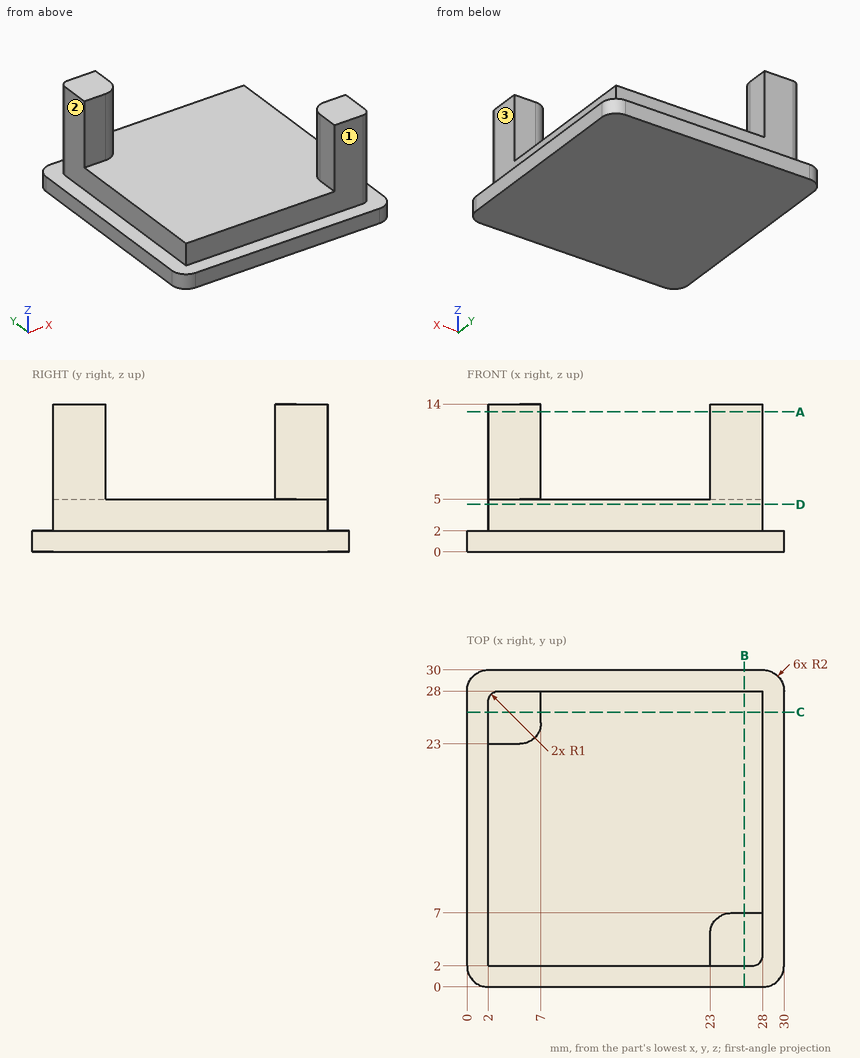
Answer from the drawing. Dimensions are ordinates in mm from the lowest x, y and z of the part. A direction names the side the tool comes from. Round coordinates to 2 decimals unless told otherwise and drop trailing zeros. Loops run counter-clockwise (first coordinate to the right, second up) from the corner with the lowest first, then second, coordinate; pieces in that order, holes last.
(1) For the marked faces 1, 2 and 3, determine the directions among +Z, -Z, +X, -X, +Y, -Y from which every point of the face is accessible in a straight line to the end or side of a thin tool.
Computed values:
face 1: +Z, +X, -X, -Y
face 2: +Z, -X, +Y, -Y
face 3: +Z, +X, +Y, -Y
(2) The part is cut by section D-D, the plane z = 4.5. Give the vertices of the cut face in (x, y).
Computed values:
outline: (2, 2) - (27, 2) arc R1 ccw to (28, 3) - (28, 28) - (3, 28) arc R1 ccw to (2, 27) - close
(3) Each of these flat-tipped pins is pushed along its axis until it touches: P1, Ø6, axis at x = 14.5, y = 10, coming from the +Z side; P2, Ø2.5, axis at x = 3, z = 11, coming from the -Y side; P3, Ø3.5, axis at y = 14.5, z = 5.5, coming from the +X side. Where does it stop, or does it pass through?
Computed values:
P1: stops at z = 5
P2: stops at y = 23
P3: stops at x = 28
(4) The part is cut by section B-B, the plane x = 26.25. Give the vertices of the cut face in (y, z), and give its area (3 significant figures).
Computed values:
outline: (0, 0) - (30, 0) - (30, 2) - (28, 2) - (28, 5) - (7, 5) - (7, 14) - (2, 14) - (2, 2) - (0, 2) - close
area: 183 mm2
(5) The part is cut by section A-A, the plane z = 13.25. Give the vertices of the cut face in (x, y).
Computed values:
outline: (2, 23) - (5, 23) arc R2 ccw to (7, 25) - (7, 28) - (3, 28) arc R1 ccw to (2, 27) - close; (23, 2) - (27, 2) arc R1 ccw to (28, 3) - (28, 7) - (25, 7) arc R2 ccw to (23, 5) - close
(6) Find the intervals of material crossed by L1, parallel to Z at x = 6, y = 11.5; L2, parallel to X at y = 26.5, z = 8.75; L3, parallel to X at y = 16.25, z = 4, in increasing order.
Computed values:
L1: z = 0 to 5
L2: x = 2 to 7
L3: x = 2 to 28
